Read the model definition and answer for the solid it produces. Units are mm, in the model's axes. A direction names the side the tool comes from. Coordinates: 2 decimals unless noted, no trailing zeros. Order: outer loops, then holes, each group sorted by start corner. A loop starts at its lowest first (then second) coordinate and runs counter-clockwise, first axis right, second up. Notation, with made-up numbers: M 22.25,82 L 69.25,82 A21 ccw 69.25,115 Z; hole C 73,21 d4. An arc over 180 degrees is marked long. Use a Markdown table: item, result. Add a question column.
1) The mould has two halves that part along X. Classify faces 4 (the face through (-8.89, 21.51, 1.48)), 5 (the face through (-6, 25, 1)), 6 (the face through (-12, 16, 1)): released by +X, released by -X, zero draft, split by the parting line, or undercut.
2) Find section B-B on x = -10. Write down the section's boundary in (y, z).
3) Find the intervals of material crossed by probe 1 along Y at (x, z) = (-10, 2.05); probe 2 along Y at (x, z) = (-1.5, 1.15); probe 3 along X at (y, z) = (13.75, 0.2), in increasing order. Write a range as [from, to].
4) Find section D-D on y = 2.5. Write down the section's boundary in (x, z), plus the area to 3 significant figures.
5) Find section C-C on z = 1.3. Write down the section's boundary in (x, y), plus the area to 3 significant figures.
6) Find section A-A on y = 20.5. Write down the section's boundary in (x, z).
7) For faces 1 (the face through (-6, 0, 1)), 2 (the face through (-32, 7.09, 1)), 3 (the face through (-20, 5, 0)), determine the directions among +Z, -Z, +X, -X, +Y, -Y from which every point of the face is accessible in a straight line to the end or side of a thin tool.
8) Each of these flat-tipped pins is pushed along its axis until it touches: pin 1 Ø1.5 at (y, z) = (12, 2) entering from -X; pin 2 Ø3.5 at (x, y) = (-10, 2.5) entering from +Z; pin 3 Ø1 at (x, z) = (-24.5, 1.5) entering from +Y; pin 4 Ø0.9 at (x, z) = (-7, 1.5) entering from -Y. Where does it stop, or does it pass through?
from build123d import *

# Parameters (mm, degrees)
SKETCH1_W           = 12
SKETCH1_H           = 25
BOSS_EXTRUDE1_DEPTH = 3
SKETCH2_R           = 1.5
CUT_EXTRUDE2_DEPTH  = 40
SKETCH4_W           = 3
SKETCH4_H           = 14.090179648
BOSS_EXTRUDE3_DEPTH = 40
SKETCH5_W           = 40
SKETCH5_H           = 3.999871266
CUT_EXTRUDE3_DEPTH  = 10


with BuildPart() as part:
    # Sketch1 → Boss-Extrude1 (new body)
    with BuildSketch(Plane.XY):
        with Locations((-6, 12.5)):
            Rectangle(SKETCH1_W, SKETCH1_H)
    extrude(amount=BOSS_EXTRUDE1_DEPTH)

    # Sketch2 → Cut-Extrude2 (cut)
    with BuildSketch(Plane(origin=(0, 0, 0), x_dir=(-1, 0, 0), z_dir=(0, 0, -1))):
        with Locations((10, 2.5)):
            Circle(SKETCH2_R)
        with Locations((10, 20.5)):
            Circle(SKETCH2_R)
    extrude(amount=-CUT_EXTRUDE2_DEPTH, mode=Mode.SUBTRACT)

    # Sketch4 → Boss-Extrude3 (add)
    with BuildSketch(Plane.ZY.offset(12)):
        with Locations((1.5, 4.045089824)):
            Rectangle(SKETCH4_W, SKETCH4_H)
    extrude(amount=BOSS_EXTRUDE3_DEPTH)

    # Sketch5 → Cut-Extrude3 (cut)
    with BuildSketch(Plane(origin=(0, 0, 0), x_dir=(-1, 0, 0), z_dir=(0, 0, -1))):
        with Locations((32, 9.090244015)):
            Rectangle(SKETCH5_W, SKETCH5_H)
    extrude(amount=-CUT_EXTRUDE3_DEPTH, mode=Mode.SUBTRACT)


solid = part.part
Check result:
| question | item | result |
|---|---|---|
| 1 | face 4 | undercut |
| 1 | face 5 | zero draft |
| 1 | face 6 | released by -X |
| 2 | outline | M 0,0 L 1,0 L 1,3 L 0,3 Z; M 4,0 L 19,0 L 19,3 L 4,3 Z; M 22,0 L 25,0 L 25,3 L 22,3 Z |
| 3 | probe 1 | y = [0, 1], [4, 19], [22, 25] |
| 3 | probe 2 | y = [0, 25] |
| 3 | probe 3 | x = [-12, 0] |
| 4 | outline | M -52,0 L -11.5,0 L -11.5,3 L -52,3 Z; M -8.5,0 L 0,0 L 0,3 L -8.5,3 Z |
| 4 | area | 147 mm2 |
| 5 | outline | M -52,-3 L -12,-3 L -12,0 L 0,0 L 0,25 L -12,25 L -12,7.09 L -52,7.09 Z; hole C -10,2.5 d3; hole C -10,20.5 d3 |
| 5 | area | 689 mm2 |
| 6 | outline | M -12,0 L -11.5,0 L -11.5,3 L -12,3 Z; M -8.5,0 L 0,0 L 0,3 L -8.5,3 Z |
| 7 | face 1 | +Z, -Z, +X, -Y |
| 7 | face 2 | +Z, -Z, -X, +Y |
| 7 | face 3 | -Z, +X, -X, +Y, -Y |
| 8 | pin 1 | stops at x = -12 |
| 8 | pin 2 | stops at z = 3 |
| 8 | pin 3 | stops at y = 7.09 |
| 8 | pin 4 | stops at y = 0 |
